Part model, mm, in its own coordinate system. A direction names the side the tool comes from. Give positions to 0.01 mm unless a question says otherwise; leave off trailing zeros. Use a Markdown table: item, result. Add a question column.
from build123d import *

# Parameters (mm, degrees)
ESQUISSE1_W                  = 10
ESQUISSE1_H                  = 10
BOSS_EXTRU_1_DEPTH           = 307
ENL_V_MAT_EXTRU_1_DEPTH      = 308.081422427
ENL_V_MAT_EXTRU_1_DEPTH_BACK = 308.081422427
ESQUISSE2_W                  = 10
ESQUISSE2_H                  = 10
ESQUISSE3_W                  = 5
ESQUISSE3_H                  = 10
ENL_V_MAT_EXTRU_2_DEPTH      = 308.203515605
D_GAGEMENT_M41_D             = 4.3
TROU_TARAUD_M3X0_51_D        = 2.5
TROU_TARAUD_M3X0_51_DEPTH    = 8.5


with BuildPart() as part:
    # Esquisse1 → Boss.-Extru.1 (new body)
    with BuildSketch(Plane.XY):
        Rectangle(ESQUISSE1_W, ESQUISSE1_H)
    extrude(amount=BOSS_EXTRU_1_DEPTH)

    # Esquisse2 → Enlèv. mat.-Extru.1 (cut, two sides: drawn at the far end of the back side and taken through both)
    with BuildSketch(Plane(origin=(0, 0, 0), x_dir=(1, 0, 0), z_dir=(0, 1, 0)).offset(-ENL_V_MAT_EXTRU_1_DEPTH_BACK)):
        with Locations((0, -5)):
            Rectangle(ESQUISSE2_W, ESQUISSE2_H)
    extrude(amount=ENL_V_MAT_EXTRU_1_DEPTH + ENL_V_MAT_EXTRU_1_DEPTH_BACK, mode=Mode.SUBTRACT)

    # Esquisse3 → Enlèv. mat.-Extru.2 (cut, through all)
    with BuildSketch(Plane.XZ.offset(5)):
        with Locations((2.5, 135)):
            Rectangle(ESQUISSE3_W, ESQUISSE3_H)
    extrude(amount=-ENL_V_MAT_EXTRU_2_DEPTH, mode=Mode.SUBTRACT)

    # Dégagement M41 (through all)
    with Locations(Plane.ZY.offset(5)):
        with Locations((86.186482928, 0), (42.586482928, 0)):
            Hole(D_GAGEMENT_M41_D / 2)

    # Trou taraudé M3x0.51
    with Locations(Plane(origin=(0, 0, 10), x_dir=(-1, 0, 0), z_dir=(0, 0, -1))):
        with Locations((0, 0)):
            Hole(TROU_TARAUD_M3X0_51_D / 2, depth=TROU_TARAUD_M3X0_51_DEPTH)


solid = part.part
1. Tool access for faces 4 (the flat face through (0, -5, 156)), 5 (the flat face through (2, 0, 130)): list every direction of +Z, -Z, +X, -X, +Y, -Y with a clear straight run to the whole face (end or side of a thin tool).
2. Mould opens along Z. For faces 1 (the flat face through (0, 0, 135)), 2 (the flat face through (-5, 0, 156)), 3 (the flat face through (-1, 1, 10)) say: released by +Z, released by -Z, zero draft, split by the parting line, or undercut.
3. Flat gauge pins, fed straight in: pin 1 (0.8 mm diameter, centred on x = 0, y = -0.5, fed in from -Z); pin 2 (3 mm diameter, centred on x = 0, y = 0, fed in from -Z); pin 3 (2.5 mm diameter, centred on y = 0, z = 86.19, fed in from -X). Where does each tip first touch, or does it go through?
4. Drill centre lines: probe 1 along Z at (x, y) = (3, 4.75); probe 2 along Y at (x, z) = (1, 86.5); probe 3 along Y at (x, z) = (0, 12.25). Where is each one in solid material? Low to high. Write a range as [from, to].
A:
| question | item | result |
|---|---|---|
| 1 | face 4 | +Z, -Z, +X, -X, -Y |
| 1 | face 5 | +X, +Y, -Y |
| 2 | face 1 | undercut |
| 2 | face 2 | zero draft |
| 2 | face 3 | released by -Z |
| 3 | pin 1 | stops at z = 18.5 |
| 3 | pin 2 | stops at z = 10 |
| 3 | pin 3 | passes through |
| 4 | probe 1 | z = [10, 130], [140, 307] |
| 4 | probe 2 | y = [-5, -2.13], [2.13, 5] |
| 4 | probe 3 | y = [-5, -1.25], [1.25, 5] |
